Can you work these out from the model? Positions are in its coordinate system, mm. Face numbers are marked on the shaded views. A direction names the side the tool comes from. Give positions to 0.01 mm unless a question says otherwise; leave off trailing zeros. Write each loop counter-clockwise with the first axis right and the second up, starting at its lowest first coordinate (ties: lowest second). Pieces come first, ordered by that corner, then holes.
from build123d import *

# Parameters (mm, degrees)
BOSS_EXTRU_1_DEPTH                                 = 5.12
CHAMBRAGE_POUR_VIS_T_TE_HEXAGONALE_M21_D           = 2
CHAMBRAGE_POUR_VIS_T_TE_HEXAGONALE_M21_CBORE_D     = 3.5
CHAMBRAGE_POUR_VIS_T_TE_HEXAGONALE_M21_CBORE_DEPTH = 1.5
CHAMBRAGE_POUR_VIS_T_TE_HEXAGONALE_M22_D           = 2
CHAMBRAGE_POUR_VIS_T_TE_HEXAGONALE_M22_CBORE_D     = 3.5
CHAMBRAGE_POUR_VIS_T_TE_HEXAGONALE_M22_CBORE_DEPTH = 1.5
CHANFREIN1_SIZE                                    = 1.3
CONG_1_R                                           = 1


with BuildPart() as part:
    # Esquisse1 → Boss.-Extru.1 (new body)
    with BuildSketch(Plane.XY):
        Polygon((0, 0), (0, 8.35), (2.8, 8.35), (2.8, 3), (8.35, 3), (8.35, 0), align=None)
    extrude(amount=BOSS_EXTRU_1_DEPTH)

    # Chambrage pour vis à tête hexagonale M21 (through all)
    with Locations(Plane(origin=(0, 3, 0), x_dir=(-1, 0, 0), z_dir=(0, 1, 0))):
        with Locations((-5.85, 2.56)):
            CounterBoreHole(CHAMBRAGE_POUR_VIS_T_TE_HEXAGONALE_M21_D / 2, CHAMBRAGE_POUR_VIS_T_TE_HEXAGONALE_M21_CBORE_D / 2, CHAMBRAGE_POUR_VIS_T_TE_HEXAGONALE_M21_CBORE_DEPTH)

    # Chambrage pour vis à tête hexagonale M22 (through all)
    with Locations(Plane.ZY):
        with Locations((2.56, 5.85)):
            CounterBoreHole(CHAMBRAGE_POUR_VIS_T_TE_HEXAGONALE_M22_D / 2, CHAMBRAGE_POUR_VIS_T_TE_HEXAGONALE_M22_CBORE_D / 2, CHAMBRAGE_POUR_VIS_T_TE_HEXAGONALE_M22_CBORE_DEPTH)

    # Chanfrein1
    chanfrein1_edges = [part.edges().sort_by_distance(p)[0] for p in [
        (0, 0, 2.56),
    ]]
    chamfer(chanfrein1_edges, length=CHANFREIN1_SIZE)

    # Congé1
    cong_1_edges = [part.edges().sort_by_distance(p)[0] for p in [
        (1.4, 8.35, 5.12),
        (1.4, 8.35, 0),
        (8.35, 1.5, 5.12),
        (8.35, 1.5, 0),
    ]]
    fillet(cong_1_edges, radius=CONG_1_R)


solid = part.part
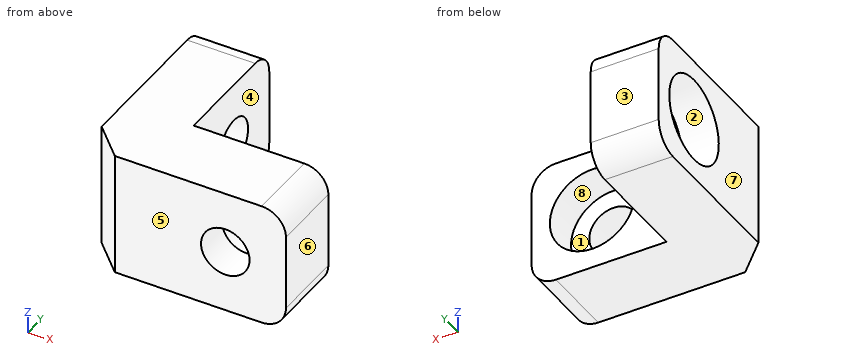
(1) If we mould it in two halves opening along X, with no side actions, what happens to the marked faces 5, 6, 7 and 8? For each: +X half, -X half, draft (parallel to the pull), parting line (faces both ways), or undercut.
Returned:
face 5: draft
face 6: +X half
face 7: -X half
face 8: undercut
(2) Imagine slicing it at C-C, the plane y = 5.85. Write out the boundary of the cut face in (x, z), plus the area to 3 significant figures.
Returned:
outline: (0, 0) - (2.8, 0) - (2.8, 1.56) - (1.5, 1.56) - (1.5, 0.81) - (0, 0.81) - close; (0, 4.31) - (1.5, 4.31) - (1.5, 3.56) - (2.8, 3.56) - (2.8, 5.12) - (0, 5.12) - close
area: 6.49 mm2
(3) If I drill on L1, parallel to Y at x = 1.9, z = 2.56; L2, parallel to Z at x = 5.85, y = 0.6; L3, parallel to Y at x = 4, z = 0.6, over which ranges is the centre line in solid material (lowest first)?
Returned:
L1: y = 0 to 4.85, 6.85 to 8.35
L2: z = 0 to 1.56, 3.56 to 5.12
L3: y = 0 to 3
(4) Imagine slicing it at B-B, the plane z = 2.56. Write out the boundary of the cut face in (x, y).
Returned:
outline: (0, 1.3) - (1.3, 0) - (4.85, 0) - (4.85, 1.5) - (4.1, 1.5) - (4.1, 3) - (2.8, 3) - (2.8, 4.85) - (1.5, 4.85) - (1.5, 4.1) - (0, 4.1) - close; (0, 7.6) - (1.5, 7.6) - (1.5, 6.85) - (2.8, 6.85) - (2.8, 8.35) - (0, 8.35) - close; (6.85, 0) - (8.35, 0) - (8.35, 3) - (7.6, 3) - (7.6, 1.5) - (6.85, 1.5) - close
(5) Imagine slicing it at D-D, the plane x = 2. Write out the boundary of the cut face in (y, z).
Returned:
outline: (0, 0) - (7.35, 0) arc R1 ccw to (8.35, 1) - (8.35, 4.12) arc R1 ccw to (7.35, 5.12) - (0, 5.12) - close; hole circle Ø2 at (5.85, 2.56)
(6) Imagine slicing it at A-A, the plane x = 5.85. Write out the boundary of the cut face in (y, z), plus the area to 3 significant figures.
Returned:
outline: (0, 0) - (3, 0) - (3, 0.81) - (1.5, 0.81) - (1.5, 1.56) - (0, 1.56) - close; (0, 3.56) - (1.5, 3.56) - (1.5, 4.31) - (3, 4.31) - (3, 5.12) - (0, 5.12) - close
area: 7.11 mm2
(7) Will these pins go through, and if not, where does the flat tip stop? P1, Ø3, axis at x = 6, z = 2, coming from the +Y side; P2, Ø2.5, axis at x = 5.85, z = 2.56, coming from the -Y side.
Returned:
P1: stops at y = 3
P2: stops at y = 0
(8) For the marked faces 1, 2, 3 and 4, which set-ups out of +Z, -Z, +X, -X, +Y, -Y let a thin tool reach every point of the face, with its end or its side?
Returned:
face 1: +Y
face 2: -X
face 3: +Z, -Z, +X, -X, +Y
face 4: +Z, -Z, +X, +Y
